Design review of the part built by this model. Coordinates are the model's own, in mm. A direction names the side the tool comes from. Coordinates: 2 decimals unless noted, no trailing zeros. Write each loop counter-clockwise with the first axis right and the second up, starting at its lowest first coordinate (ties: lowest second). Pieces come first, ordered by that corner, then holes.
Q1. Insertion check: pin 1 (25 mm diameter, centred on x = -52.5, z = -32, fed in from -Y); pin 2 (12 mm diameter, centred on x = 28, y = -163, fed in from -Z); pin 3 (3 mm diameter, centred on x = -6.5, z = 15, fed in from +Y). Each pin has a flat end and moves straight along its axis. Give the tip position at first contact, or say it passes through.
Q2. For probe 1 along Y at (x, z) = (59.5, -88); probe 2 along Y at (x, z) = (-61, -91); probe 3 along X at (y, z) = (-142, 32), list the stretches that pass through material, from the lowest coordinate up.
Q3. Take a section at B-B (z = 9). Give the boundary of the cut face in (x, y), and give its area (3 significant figures).
Q4. Take a section at D-D (z = 52.5). Give the boundary of the cut face in (x, y).
Q5. Mouldability with a two-part tool opening along Z and no side actions: class faces 4 (the flat face through (87.3, -153, 46)), 5 (the cylindrical face through (23.93, -56.35, -93.74)), 6 (the flat face through (52, -148, 87.3)) as pulls with the +Z half, pulls with the -Z half, needs draft (parallel to the pull), parting line crosses it, or undercut.
Q6. Take a section at A-A (x = 0). Give the boundary of the cut face in (y, z).
Q7. Machinability: for faces 1 (the flat face through (-57, -46, 87.3)), 2 (the flat face through (42, -40, -87.3)), 3 (the flat face through (87.3, -54, -38)), which of the approach directions +Z, -Z, +X, -X, +Y, -Y give a long, thin tool a straight path to every point of the face, cutting with its end or side? Answer none if there is none.
```python
from build123d import *

# Parameters (mm, degrees)
F0_W         = 200
F0_H         = 200
F1_DEPTH     = 200
F2_R         = 12.7
F3_T1_DEPTH  = 206.35
F3_T3_DEPTH  = 174.6
F3_T5_DEPTH  = 206.35
F3_S9_W      = 12.954
F3_S9_H      = 12.954
F3_T10_DEPTH = 12.954
F3_S15_W     = 12.954
F3_S15_H     = 12.954
F3_T16_DEPTH = 12.954
F4_R         = 25
F5_DEPTH     = 12.7
F6_R         = 25
F7_DEPTH     = 12.7
F8_DEPTH     = 12.7
F9_R         = 25
F10_DEPTH    = 12.7
F11_R        = 25
F12_DEPTH    = 12.7
F13_R        = 25
F14_DEPTH    = 12.7
F15_R        = 25
F16_DEPTH    = 12.7


# Not quite as in the source:
# - a fillet or chamfer that OpenCascade refuses, or shapes differently, is made with other operations: its cross-section is extruded or revolved along the edge and cut away or added


with BuildPart() as f1:
    # F0 (on Front) → F1 (new body)
    with BuildSketch(Plane.XZ):
        Rectangle(F0_W, F0_H)
    extrude(amount=F1_DEPTH)

    # F2
    f2_edges = [f1.edges().sort_by_distance(p)[0] for p in [
        (100, -100, -100),
        (100, -100, 100),
        (100, 0, 0),
        (100, -200, 0),
        (0, -200, -100),
        (0, -200, 100),
        (-100, -200, 0),
    ]]
    fillet(f2_edges, radius=F2_R)

    # F3: fillet of radius 12.7 on 11 edges, made by hand

    # F3_s2 → F3_t1 (cut)
    with BuildSketch(Plane.XZ.offset(12.7)):
        with BuildLine():
            ThreePointArc((-100, 87.3), (-96.2802561211, 96.2802561211), (-87.3, 100))
            Line((-87.3, 100), (-100, 100))
            Line((-100, 100), (-100, 87.3))
        make_face()
        with BuildLine():
            ThreePointArc((-87.3, -100), (-96.2802561211, -96.2802561211), (-100, -87.3))
            Line((-100, -87.3), (-100, -100))
            Line((-100, -100), (-87.3, -100))
        make_face()
    extrude(amount=F3_T1_DEPTH, mode=Mode.SUBTRACT)

    # F3_s4 → F3_t3 (cut)
    with BuildSketch(Plane.XY.offset(-87.3)):
        with BuildLine():
            ThreePointArc((-100, -12.7), (-96.2802561211, -3.7197438789), (-87.3, 0))
            Line((-87.3, 0), (-100, 0))
            Line((-100, 0), (-100, -12.7))
        make_face()
    extrude(amount=F3_T3_DEPTH, mode=Mode.SUBTRACT)

    # F3_s6 → F3_t5 (cut)
    with BuildSketch(Plane.YZ.offset(-87.3)):
        with BuildLine():
            ThreePointArc((0, 87.3), (-3.7197438789, 96.2802561211), (-12.7, 100))
            Line((-12.7, 100), (0, 100))
            Line((0, 100), (0, 87.3))
        make_face()
        with BuildLine():
            ThreePointArc((-12.7, -100), (-3.7197438789, -96.2802561211), (0, -87.3))
            Line((0, -87.3), (0, -100))
            Line((0, -100), (-12.7, -100))
        make_face()
    extrude(amount=F3_T5_DEPTH, mode=Mode.SUBTRACT)


with BuildPart() as f3_tool8:
    # F3_s9 → F3_t10 (new body)
    with BuildSketch(Plane.YZ.offset(-87.3)):
        with Locations((-6.223, 93.777)):
            Rectangle(F3_S9_W, F3_S9_H)
    extrude(amount=-F3_T10_DEPTH)

    # F3_s11 → F3_t12 (revolve, cut)
    with BuildSketch(Plane(origin=(-87.3, -12.7, 87.3), x_dir=(0, -0.7071067812, -0.7071067812), z_dir=(0, 0.7071067812, -0.7071067812))):
        with BuildLine():
            ThreePointArc((0, -12.7), (12.7, 0), (0, 12.7))
            Line((0, 12.7), (0, -12.7))
        make_face()
    revolve(axis=Axis((-87.3, -12.7, 87.3), (-1, 0, 0)), mode=Mode.SUBTRACT)


with BuildPart() as f1_1:
    add(f1.part)

    # F3_t7: cut F3_tool8
    add(f3_tool8.part, mode=Mode.SUBTRACT)


with BuildPart() as f3_tool14:
    # F3_s15 → F3_t16 (new body)
    with BuildSketch(Plane.XY.offset(-87.3)):
        with Locations((-93.777, -6.223)):
            Rectangle(F3_S15_W, F3_S15_H)
    extrude(amount=-F3_T16_DEPTH)

    # F3_s17 → F3_t18 (revolve, cut)
    with BuildSketch(Plane(origin=(-87.3, -12.7, -87.3), x_dir=(0.7071067812, -0.7071067812, 0), z_dir=(0.7071067812, 0.7071067812, 0))):
        with BuildLine():
            ThreePointArc((0, -12.7), (12.7, 0), (0, 12.7))
            Line((0, 12.7), (0, -12.7))
        make_face()
    revolve(axis=Axis((-87.3, -12.7, -87.3), (0, 0, -1)), mode=Mode.SUBTRACT)


with BuildPart() as f1_2:
    add(f1_1.part)

    # F3_t13: cut F3_tool14
    add(f3_tool14.part, mode=Mode.SUBTRACT)

    # F4 (on face) → F5 (cut)
    with BuildSketch(Plane(origin=(0, 0, 0), x_dir=(-1, 0, 0), z_dir=(0, 1, 0))):
        Circle(F4_R)
    extrude(amount=-F5_DEPTH, mode=Mode.SUBTRACT)

    # F6 (on face) → F7 (cut)
    with BuildSketch(Plane.XY.offset(100)):
        with Locations((-56.3085600734, -46.6261841357)):
            Circle(F6_R)
        with Locations((52.2117828626, -148.8133593049)):
            Circle(F6_R)
    extrude(amount=-F7_DEPTH, mode=Mode.SUBTRACT)

    # F6 (on face) → F8 (cut)
    with BuildSketch(Plane.XY.offset(100)):
        with Locations((-56.3085600734, -46.6261841357)):
            Circle(F6_R)
        with Locations((52.2117828626, -148.8133593049)):
            Circle(F6_R)
    extrude(amount=-F8_DEPTH, mode=Mode.SUBTRACT)

    # F9 (on face) → F10 (cut)
    with BuildSketch(Plane.YZ.offset(100)):
        with Locations((-152.8625637293, 45.855615288)):
            Circle(F9_R)
        with Locations((-104.9481332302, 6.1764707789)):
            Circle(F9_R)
        with Locations((-53.6647066474, -38.3689813316)):
            Circle(F9_R)
    extrude(amount=-F10_DEPTH, mode=Mode.SUBTRACT)

    # F11 (on face) → F12 (cut)
    with BuildSketch(Plane(origin=(-100, 0, 0), x_dir=(0, -1, 0), z_dir=(-1, 0, 0))):
        with Locations((50.6975390017, -48.2849427062)):
            Circle(F11_R)
        with Locations((48.2081025839, 42.5794422626)):
            Circle(F11_R)
        with Locations((144.8811888695, 41.3347259164)):
            Circle(F11_R)
        with Locations((148.2004225254, -47.8700399399)):
            Circle(F11_R)
    extrude(amount=-F12_DEPTH, mode=Mode.SUBTRACT)

    # F13 (on face) → F14 (cut)
    with BuildSketch(Plane.XZ.offset(200)):
        with Locations((-56.1834387481, 45.481286943)):
            Circle(F13_R)
        with Locations((-56.5915383924, -43.1586373624)):
            Circle(F13_R)
        with Locations((56.8646900356, -45.1069548726)):
            Circle(F13_R)
        with Locations((54.9930334091, 45.8556227386)):
            Circle(F13_R)
        Circle(F13_R)
    extrude(amount=-F14_DEPTH, mode=Mode.SUBTRACT)

    # F15 (on face) → F16 (cut)
    with BuildSketch(Plane(origin=(0, 0, -100), x_dir=(1, 0, 0), z_dir=(0, 0, -1))):
        with Locations((-53.2460398972, 155.2098095417)):
            Circle(F15_R)
        with Locations((-53.4454273642, 99.2308959943)):
            Circle(F15_R)
        with Locations((-54.8167897346, 40.5999273626)):
            Circle(F15_R)
        with Locations((39.449018472, 157.1737299708)):
            Circle(F15_R)
        with Locations((40.3425594879, 98.5919412215)):
            Circle(F15_R)
        with Locations((42.359188109, 39.4558809987)):
            Circle(F15_R)
    extrude(amount=-F16_DEPTH, mode=Mode.SUBTRACT)


solid = f1_2.part
```
Response:
1. pin 1: stops at y = -187.3
1. pin 2: stops at z = -87.3
1. pin 3: stops at y = -12.7
2. probe 1: y = -199.98 to -172.11, -142.24 to -114.65, -82.53 to -57.65, -21.26 to -0.02
2. probe 2: y = -199.45 to -178.98, -131.44 to -123.06, -75.4 to -64.82, -16.38 to -0.55
2. probe 3: x = -87.3 to 87.3
3. outline: (-100, -187.3) arc R12.7 ccw to (-87.3, -200) - (-23.32, -200) - (-23.32, -187.3) - (23.32, -187.3) - (23.32, -200) - (87.3, -200) arc R12.7 ccw to (100, -187.3) - (100, -129.79) - (87.3, -129.79) - (87.3, -80.11) - (100, -80.11) - (100, -12.7) arc R12.7 ccw to (87.3, 0) - (23.32, 0) - (23.32, -12.7) - (-23.32, -12.7) - (-23.32, 0) - (-87.3, 0) arc R12.7 ccw to (-100, -12.7) - close
3. area: 38,000 mm2
4. outline: (-100, -187.3) arc R12.7 ccw to (-87.3, -200) - (-80.18, -200) - (-80.18, -187.3) - (-32.19, -187.3) - (-32.19, -200) - (30.89, -200) - (30.89, -187.3) - (79.09, -187.3) - (79.09, -200) - (87.3, -200) arc R12.7 ccw to (100, -187.3) - (100, -176.96) - (87.3, -176.96) - (87.3, -128.76) - (100, -128.76) - (100, -12.7) arc R12.7 ccw to (87.3, 0) - (-87.3, 0) arc R12.7 ccw to (-100, -12.7) - (-100, -25.26) - (-87.3, -25.26) - (-87.3, -71.16) - (-100, -71.16) - (-100, -122.51) - (-87.3, -122.51) - (-87.3, -167.25) - (-100, -167.25) - close
5. face 4: undercut
5. face 5: needs draft
5. face 6: pulls with the +Z half
6. outline: (-200, -87.3) arc R12.7 ccw to (-187.3, -100) - (-12.7, -100) arc R12.7 ccw to (0, -87.3) - (0, -25) - (-12.7, -25) - (-12.7, 25) - (0, 25) - (0, 87.3) arc R12.7 ccw to (-12.7, 100) - (-187.3, 100) arc R12.7 ccw to (-200, 87.3) - (-200, 25) - (-187.3, 25) - (-187.3, -25) - (-200, -25) - close
7. face 1: +Z
7. face 2: -Z
7. face 3: +X
